Check sheet for the drawn part. Datum: minimum x, y, z corner. Units: mm. A direction names the side the tool comes from. Round coordinates to 2 decimals unless told otherwise and drop trailing zeros. Write each loop counter-clockwise with the first axis right and the second up, starting at its lowest first coordinate (ties: lowest second). Pieces come first, ordered by that corner, then holes. Notation, with made-up numbers: (62.25, 0.25) - (111.25, 0.25) arc R23 ccw to (111.25, 8.25) - close; hole circle Ø9 at (-3, 86). An arc over 180 degrees is marked (long way). Answer as a JSON object with one key per item and string values. Group by question number.
1) Go/stop test with flat-tipped pins: pin 1 Ø3 at (y, z) = (3, 24.5) entering from -X; pin 2 Ø9 at (x, z) = (78, 18) entering from -Y (3 decimals); pin 3 Ø15 at (x, z) = (50.5, 15.5) entering from +Y (3 decimals). Record where each tip stops, or that it passes through.
2) Section check A-A (y = 11). Enter the section's corners in (x, z).
3) Section check C-C (x = 12). Enter the section's corners in (y, z).
4) Section check B-B (z = 7.5). Enter the section's corners in (x, y) (1 decimal).
5) Mould release check, pull along Y, two halves, no side actions. Record for the marked faces 4, 5, 6 and 7: +Y half, -Y half, draft (parallel to the pull), parting line (faces both ways), or undercut.
6) Thickness scan on line 1 (Y direction, x = 54, z = 2.5) (1 decimal); line 2 (X direction, y = 9.75, z = 24.75) (1 decimal); line 3 (X direction, y = 12.75, z = 24.5) (1 decimal). Record the ranges inside material, lowest first.
7) Set-up check for the marked faces 1, 2 and 3: record each of +Z, -Z, +X, -X, +Y, -Y from which the full face is reachable in a straight line by a thin tool's end or side.
8) Section check D-D (z = 16.25). Enter the section's corners in (x, y) (1 decimal), then the cut area to 3 significant figures.
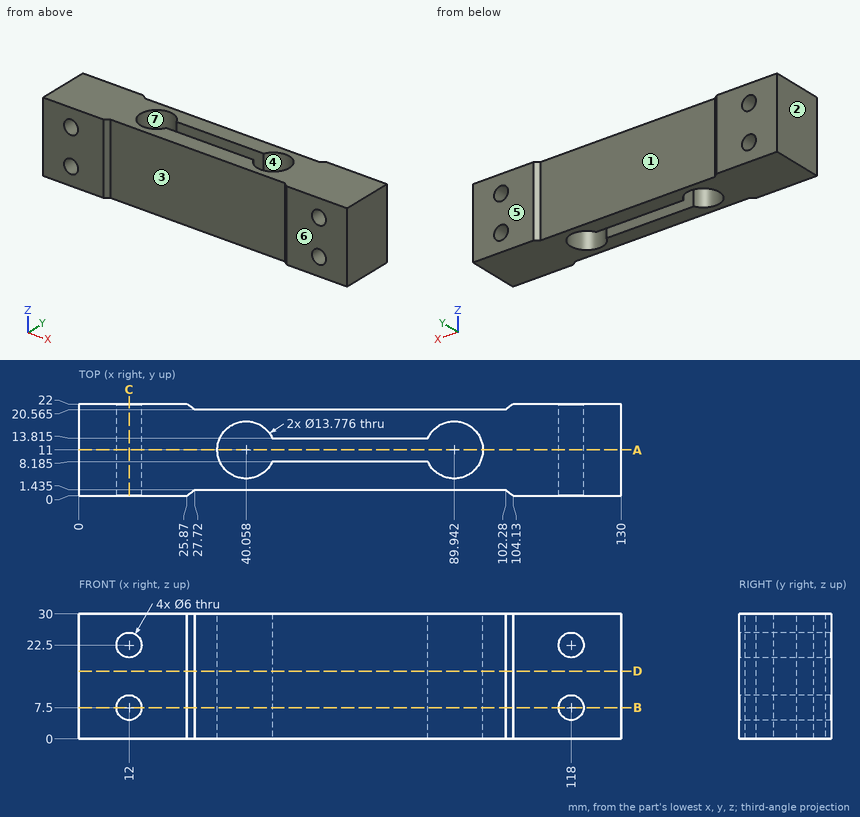
Returned:
{
 "1": {"pin 1": "x = 0", "pin 2": "y = 1.435", "pin 3": "y = 20.565"},
 "2": {"outline": "(0, 0) - (33.17, 0) - (33.17, 30) - (0, 30) - close; (96.83, 0) - (130, 0) - (130, 30) - (96.83, 30) - close; hole circle Ø6 at (12, 7.5); hole circle Ø6 at (12, 22.5); hole circle Ø6 at (118, 7.5); hole circle Ø6 at (118, 22.5)"},
 "3": {"outline": "(0, 0) - (22, 0) - (22, 4.5) - (0, 4.5) - close; (0, 10.5) - (22, 10.5) - (22, 19.5) - (0, 19.5) - close; (0, 25.5) - (22, 25.5) - (22, 30) - (0, 30) - close"},
 "4": {"outline": "(0, 0) - (9, 0) - (9, 22) - (0, 22) - close; (15, 0) - (25.9, 0) - (27.7, 1.4) - (102.3, 1.4) - (104.1, 0) - (115, 0) - (115, 22) - (104.1, 22) - (102.3, 20.6) - (27.7, 20.6) - (25.9, 22) - (15, 22) - close; (121, 0) - (130, 0) - (130, 22) - (121, 22) - close; hole (46.3, 8.2) - (83.7, 8.2) arc R6.9 ccw (long way) to (83.7, 13.8) - (46.3, 13.8) arc R6.9 ccw (long way) to start"},
 "5": {"face 4": "undercut", "face 5": "+Y half", "face 6": "-Y half", "face 7": "undercut"},
 "6": {"line 1": "1.4 to 8.2, 13.8 to 20.6", "line 2": "0 to 10, 14 to 33.3, 96.7 to 116, 120 to 130", "line 3": "0 to 9.8, 14.2 to 33.4, 96.6 to 115.8, 120.2 to 130"},
 "7": {"face 1": "+Z, -Z, +Y", "face 2": "+Z, -Z, -X, +Y, -Y", "face 3": "+Z, -Z, -Y"},
 "8": {"outline": "(0, 0) - (25.9, 0) - (27.7, 1.4) - (102.3, 1.4) - (104.1, 0) - (130, 0) - (130, 22) - (104.1, 22) - (102.3, 20.6) - (27.7, 20.6) - (25.9, 22) - (0, 22) - close; hole (46.3, 8.2) - (83.7, 8.2) arc R6.9 ccw (long way) to (83.7, 13.8) - (46.3, 13.8) arc R6.9 ccw (long way) to start", "area": "2,140 mm2"}
}
